Could you check a few things on this drawing? It's one solid part, dimensions in mm from its lowest x, y, z. Coordinates: 2 decimals unless noted, no trailing zeros. Order: outer loops, then holes, each group sorted by start corner. A loop starts at its lowest first (then second) coordinate and runs counter-clockwise, first axis right, second up. Notation, with made-up numbers: (26.25, 78.25) - (52.25, 78.25) arc R15 ccw to (52.25, 90.25) - close; hole circle Ø10 at (61, -34.75). An arc over 180 degrees is marked (long way). Return JSON: item names as keys, results as strings. Group by question number.
1) Imagine slicing it at C-C (z = 2.55). Write out the boundary of the cut face in (x, y) (3 decimals), and give its area (3 significant figures).
2) If I drill on line 1 along Y through (x, z) = (52.5, 2.1) (3 decimals); line 2 along X through (y, z) = (2.75, 0.8); line 3 along X through (y, z) = (6.25, 3.7), over which ranges is the centre line in solid material (lowest first)?
3) Imagine slicing it at A-A (y = 5). Write out the boundary of the cut face in (x, z) (3 decimals).
4) Imagine slicing it at B-B (x = 52.5). Write out the boundary of the cut face in (y, z) (3 decimals), and give its area (4 significant figures).
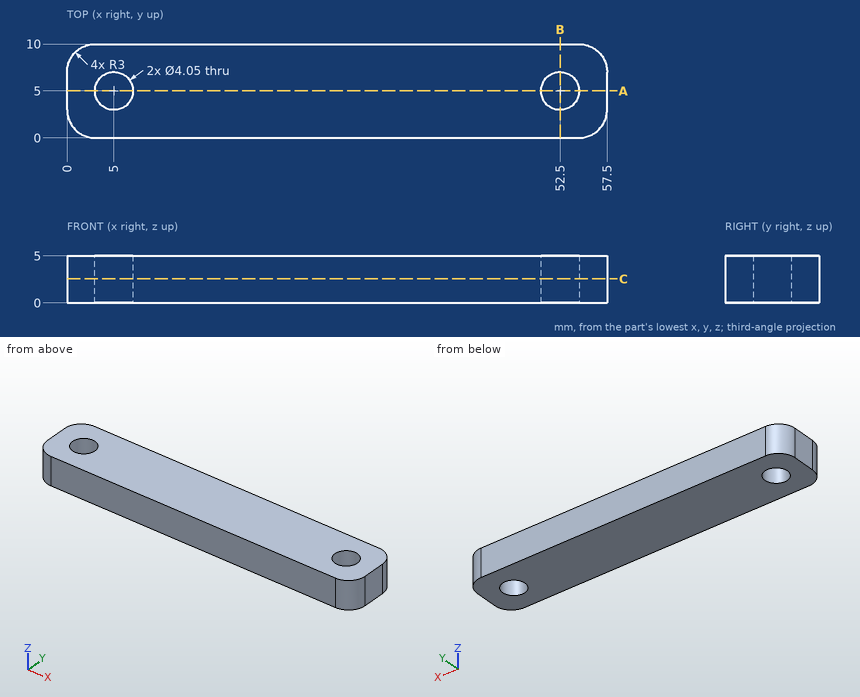
Calculated:
{
 "1": {"outline": "(0, 3) arc R3 ccw to (3, 0) - (54.5, 0) arc R3 ccw to (57.5, 3) - (57.5, 7) arc R3 ccw to (54.5, 10) - (3, 10) arc R3 ccw to (0, 7) - close; hole circle Ø4.05 at (5, 5); hole circle Ø4.05 at (52.5, 5)", "area": "542 mm2"},
 "2": {"line 1": "0 to 2.975, 7.025 to 10", "line 2": "0.01 to 57.49", "line 3": "0 to 3.41, 6.59 to 50.91, 54.09 to 57.5"},
 "3": {"outline": "(0, 0) - (2.975, 0) - (2.975, 5) - (0, 5) - close; (7.025, 0) - (50.475, 0) - (50.475, 5) - (7.025, 5) - close; (54.525, 0) - (57.5, 0) - (57.5, 5) - (54.525, 5) - close"},
 "4": {"outline": "(0, 0) - (2.975, 0) - (2.975, 5) - (0, 5) - close; (7.025, 0) - (10, 0) - (10, 5) - (7.025, 5) - close", "area": "29.75 mm2"}
}
